Part model, mm, in its own coordinate system. A direction names the side the tool comes from. Round coordinates to 2 decimals unless told otherwise and drop trailing zeros. Write each loop counter-clockwise with the first axis right and the second up, starting at its lowest first coordinate (ties: lowest second). Pieces come first, ordered by that corner, then holes.
```python
from build123d import *

# Parameters (mm, degrees)
SKETCH1_W           = 2500
SKETCH1_H           = 1480
BOSS_EXTRUDE1_DEPTH = 100
SHELL1_T            = -20
FILLET1_R           = 10


with BuildPart() as part:
    # Sketch1 → Boss-Extrude1 (new body)
    with BuildSketch(Plane.XY):
        with Locations((1250, 740)):
            Rectangle(SKETCH1_W, SKETCH1_H)
    extrude(amount=BOSS_EXTRUDE1_DEPTH)

    # Shell1
    shell1_openings = [part.faces().sort_by_distance(p)[0] for p in [
        (1250, 740, 0),
    ]]
    offset(amount=SHELL1_T, openings=shell1_openings, kind=Kind.INTERSECTION)

    # Fillet1
    fillet1_edges = [part.edges().sort_by_distance(p)[0] for p in [
        (2500, 740, 100),
        (1250, 1480, 100),
        (0, 740, 100),
        (0, 1480, 50),
        (2500, 1480, 50),
        (2500, 0, 50),
        (0, 0, 50),
        (1250, 0, 100),
    ]]
    fillet(fillet1_edges, radius=FILLET1_R)


solid = part.part
```
Q1. Cut at A-A on x = 1903.5. Write the cut outline in (y, z), plus the area to 3 significant figures.
Values follow:
outline: (0, 0) - (20, 0) - (20, 80) - (1460, 80) - (1460, 0) - (1480, 0) - (1480, 90) arc R10 ccw to (1470, 100) - (10, 100) arc R10 ccw to (0, 90) - close
area: 32,800 mm2
Q2. Wall check: L1, parallel to Y at x = 429, z = 33; L2, parallel to X at y = 265, z = 51; L3, parallel to Z at x = 2030.5, y = 1222. Give the ranges that are in metal, low to high.
Values follow:
L1: y = 0 to 20, 1460 to 1480
L2: x = 0 to 20, 2480 to 2500
L3: z = 80 to 100
Q3. Cut at B-B on y = 415. Write the cut outline in (x, z), plus the area to 3 significant figures.
Values follow:
outline: (0, 0) - (20, 0) - (20, 80) - (2480, 80) - (2480, 0) - (2500, 0) - (2500, 90) arc R10 ccw to (2490, 100) - (10, 100) arc R10 ccw to (0, 90) - close
area: 53,200 mm2
Q4. Cut at C-C on z = 56. Write the cut outline in (x, y), plus the area to 3 significant figures.
Values follow:
outline: (0, 10) arc R10 ccw to (10, 0) - (2490, 0) arc R10 ccw to (2500, 10) - (2500, 1470) arc R10 ccw to (2490, 1480) - (10, 1480) arc R10 ccw to (0, 1470) - close; hole (20, 20) - (2480, 20) - (2480, 1460) - (20, 1460) - close
area: 158,000 mm2
Q5. Which spindle directions (+Z, -Z, +X, -X, +Y, -Y) get a long thin tool onto all of the face, cutting with end or side? Do faces 5 (the flat face through (1233, 0, 44)), 6 (the flat face through (1233, 1460, 39)). Say none if no direction does.
Values follow:
face 5: +Z, -Z, +X, -X, -Y
face 6: -Z
Q6. Mould opens along X. For faces 1 (the flat face through (1233, 750, 80)), 2 (the flat face through (0, 730, 44)), 3 (the flat face through (1233, 750, 100)), 4 (the flat face through (2500, 730, 44)) say: +X half, -X half, draft (parallel to the pull), parting line (faces both ways), or undercut.
Values follow:
face 1: undercut
face 2: -X half
face 3: draft
face 4: +X half
